The drawing under review shows one solid part. Ordinate dimensions are in mm from its lowest x, y, z. A direction names the side the tool comes from. Give positions to 0.01 mm unless a question says otherwise; leave off trailing zeros. Write each loop counter-clockwise with the first axis right and the second up, starting at its lowest first coordinate (ties: lowest second). Pieces come first, ordered by that corner, then holes. Notation, with made-up numbers: M 81,3.25 L 115,3.25 A17 ccw 115,26.25 Z; hole C 33.5,-33.5 d9. An arc over 180 degrees is marked long. Answer as a JSON object with one key per item and string values. Group by question number.
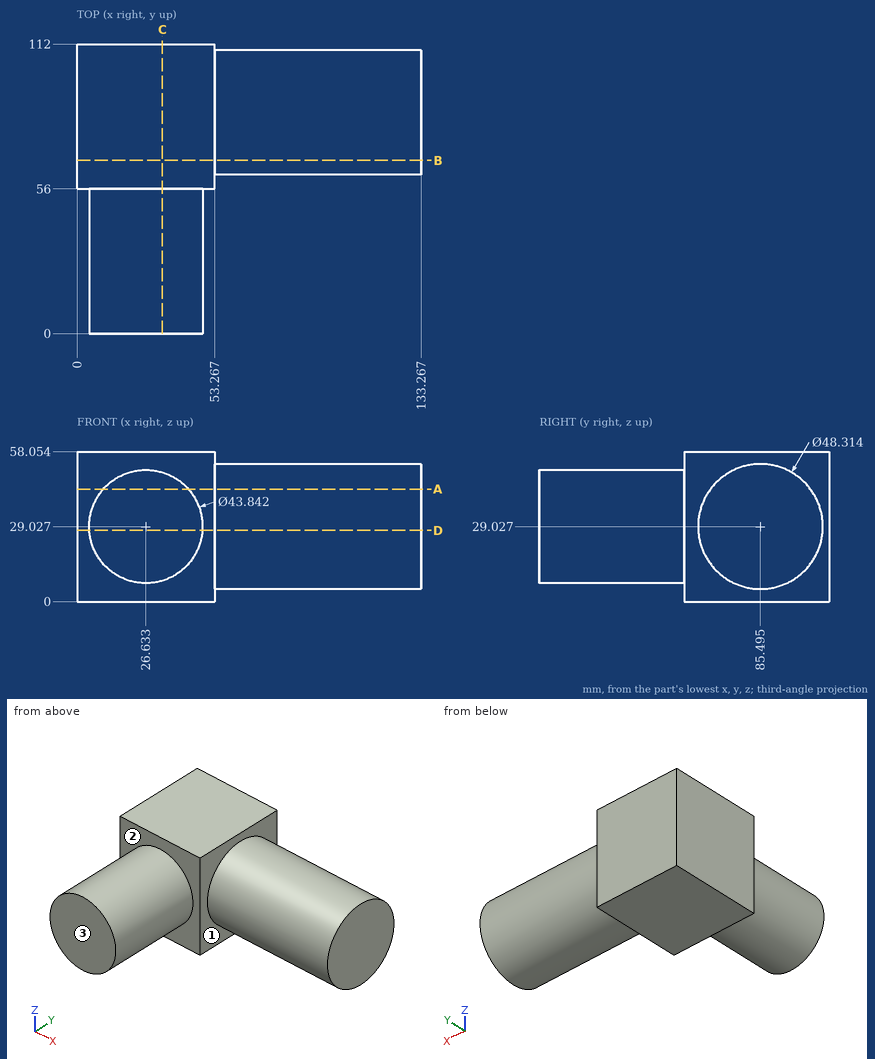
Item 1: Consider section D-D (z = 27.5). Give the boundary of the cut face in (x, y) (1 decimal), plus the area to 3 significant figures.
Item 2: To check wall thickness, follow probe 1 along X at (y, z) = (105.5, 53); probe 2 along Z at (x, y) = (106, 86) (1 decimal); probe 3 along Y at (x, z) = (39, 2.5). State the ranges of each line that lie inside material, in increasing order.
Item 3: Consider section B-B (y = 67). Give the boundary of the cut face in (x, z), plus the area to 3 significant figures.
Item 4: Consider section C-C (x = 33). Give the boundary of the cut face in (y, z).
Item 5: Consider section A-A (z = 43.5). Give the boundary of the cut face in (x, y) (1 decimal).
Item 6: Machinability: for the marked faces 1, 2 and 3, which of the approach directions +Z, -Z, +X, -X, +Y, -Y give a long, thin tool a straight path to every point of the face, cutting with its end or side? Answer none if there is none.
Item 7: Insertion check: P1, Ø3, axis at x = 116, z = 40.5, coming from the -Y side; P2, Ø3, axis at x = 91, y = 86, coming from the -Z side; P3, Ø8, axis at x = 100.5, z = 46, coming from the -Y side; P4, Ø12, axis at y = 57.5, z = 20.5, coming from the -X side. Each pin has a flat end and moves straight along its axis. Give the tip position at first contact, or say it passes through.
Result set:
{
 "1": {"outline": "M 0,56 L 4.8,56 L 4.8,0 L 48.5,0 L 48.5,56 L 53.3,56 L 53.3,61.4 L 133.3,61.4 L 133.3,109.6 L 53.3,109.6 L 53.3,112 L 0,112 Z", "area": "9,290 mm^2"},
 "2": {"probe 1": "x = 0 to 53.27", "probe 2": "z = 4.9 to 53.2", "probe 3": "y = 56 to 112"},
 "3": {"outline": "M 0,0 L 53.27,0 L 53.27,13.49 L 133.27,13.49 L 133.27,44.57 L 53.27,44.57 L 53.27,58.05 L 0,58.05 Z", "area": "5,580 mm^2"},
 "4": {"outline": "M 0,8.05 L 56,8.05 L 56,0 L 112,0 L 112,58.05 L 56,58.05 L 56,50 L 0,50 Z"},
 "5": {"outline": "M 0,56 L 10.2,56 L 10.2,0 L 43.1,0 L 43.1,56 L 53.3,56 L 53.3,66.2 L 133.3,66.2 L 133.3,104.8 L 53.3,104.8 L 53.3,112 L 0,112 Z"},
 "6": {"face 1": "+X", "face 2": "-Y", "face 3": "+Z, -Z, +X, -X, -Y"},
 "7": {"P1": "stops at y = 63.49", "P2": "stops at z = 4.87", "P3": "stops at y = 65.12", "P4": "stops at x = 0"}
}
